Input: part model. Units: mm. Frame: model coordinates. A direction names the side the tool comes from. Round coordinates to 2 decimals unless told otherwise and drop trailing zeros. Write each loop counter-clockwise with the first axis right and the second up, starting at its lowest first coordinate (ties: lowest second). Pieces come first, ordered by that corner, then holes. Notation, with made-up numbers: (29.25, 63.25) -> (53.25, 63.25) arc R18 cw to (53.25, 73.25) -> close; hole circle Ø7 at (26, -17.5). An arc over 180 degrees is marked (long way). Write item = value, one per line.
```python
from build123d import *

# Parameters (mm, degrees)
SKETCH1_W                  = 38.1
SKETCH1_H                  = 88.9
BOSS_BASE_DEPTH            = 2.286
SKETCH3_W                  = 38.1
SKETCH3_H                  = 2.1717
BOSS_LIP_DEPTH             = 23.25116
F_4_0_209_DIAMETER_HOLE1_D = 5.3086
F_4_0_209_DIAMETER_HOLE2_D = 5.3086
SKETCH19_W                 = 4.445
SKETCH19_H                 = 66.04
CUT_EXTRUDE1_DEPTH         = 54.659308991
FILLET1_R                  = 3.81
FILLET4_R                  = 0.635


with BuildPart() as part:
    # Sketch1 → Boss-Base (new body)
    with BuildSketch(Plane(origin=(0, 0, 0), x_dir=(1, 0, 0), z_dir=(0, 1, 0))):
        Rectangle(SKETCH1_W, SKETCH1_H)
    extrude(amount=BOSS_BASE_DEPTH)

    # Sketch3 → Boss-Lip (add)
    with BuildSketch(Plane(origin=(0, 2.286, 0), x_dir=(1, 0, 0), z_dir=(0, 1, 0))):
        with Locations((0, 43.36415)):
            Rectangle(SKETCH3_W, SKETCH3_H)
    extrude(amount=BOSS_LIP_DEPTH)

    # #4 (0.209) Diameter Hole1 (through all)
    with Locations(Plane(origin=(0, 2.286, 0), x_dir=(1, 0, 0), z_dir=(0, 1, 0))):
        with Locations((0, -33.9217), (0, 6.7183)):
            Hole(F_4_0_209_DIAMETER_HOLE1_D / 2)

    # #4 (0.209) Diameter Hole2 (through all)
    with Locations(Plane.XY.offset(-42.2783)):
        with Locations((10.16, 17.78), (-10.16, 17.78)):
            Hole(F_4_0_209_DIAMETER_HOLE2_D / 2)

    # Sketch19 → Cut-Extrude1 (cut, through all)
    with BuildSketch(Plane(origin=(0, 2.286, 0), x_dir=(1, 0, 0), z_dir=(0, 1, 0))):
        with Locations((16.8275, -11.43)):
            Rectangle(SKETCH19_W, SKETCH19_H)
        with Locations((-16.8275, -11.43)):
            Rectangle(SKETCH19_W, SKETCH19_H)
    extrude(amount=-CUT_EXTRUDE1_DEPTH, mode=Mode.SUBTRACT)

    # Fillet1
    fillet1_edges = [part.edges().sort_by_distance(p)[0] for p in [
        (0, 2.286, -42.2783),
        (-19.05, 25.53716, -43.36415),
        (19.05, 25.53716, -43.36415),
        (0, 0, -44.45),
        (19.05, 1.143, -21.59),
        (14.605, 1.143, 44.45),
        (-19.05, 1.143, -21.59),
        (-14.605, 1.143, 44.45),
    ]]
    fillet(fillet1_edges, radius=FILLET1_R)

    # Fillet4
    fillet4_edges = [part.edges().sort_by_distance(p)[0] for p in [
        (19.05, 1.115923164, -43.334076836),
        (19.05, 3.401923164, -41.162376836),
        (-19.05, 3.401923164, -41.162376836),
        (14.605, 0, 9.525),
        (14.605, 2.286, 9.525),
        (-14.9225, 0, -21.59),
        (-14.9225, 2.286, -21.59),
        (19.05, 13.91158, -42.2783),
        (0, 25.53716, -42.2783),
        (-19.05, 13.91158, -42.2783),
        (17.934076836, 24.421236836, -42.2783),
        (-17.934076836, 24.421236836, -42.2783),
        (14.9225, 2.286, -21.59),
        (19.05, 2.286, -31.93415),
        (-19.05, 2.286, -31.93415),
        (-14.605, 2.286, 9.525),
        (0, 2.286, 44.45),
        (-17.934076836, 2.286, -22.705923164),
        (17.934076836, 2.286, -22.705923164),
        (13.489076836, 2.286, 43.334076836),
        (-13.489076836, 2.286, 43.334076836),
        (-19.05, 12.76858, -44.45),
        (0, 25.53716, -44.45),
        (19.05, 12.76858, -44.45),
        (17.934076836, 24.421236836, -44.45),
        (-17.934076836, 24.421236836, -44.45),
        (-19.05, 0, -33.02),
        (-19.05, 1.115923164, -43.334076836),
        (14.9225, 0, -21.59),
        (0, 0, 44.45),
        (-14.605, 0, 9.525),
        (19.05, 0, -33.02),
        (-17.934076836, 0, -22.705923164),
        (17.934076836, 0, -22.705923164),
        (13.489076836, 0, 43.334076836),
        (-13.489076836, 0, 43.334076836),
    ]]
    fillet(fillet4_edges, radius=FILLET4_R)


solid = part.part
```
1) Cut plane D-D (y = 7.25). Return the cut outline in (x, z) (3 decimals).
Solutions:
outline = (-19.05, -43.815) arc R0.635 ccw to (-18.415, -44.45) -> (18.415, -44.45) arc R0.635 ccw to (19.05, -43.815) -> (19.05, -42.913) arc R0.635 ccw to (18.415, -42.278) -> (-18.415, -42.278) arc R0.635 ccw to (-19.05, -42.913) -> close
2) First-contact query: P1, Ø0.5, axis at x = -15, y = 1.5, coming from the +Z side; P2, Ø0.5, axis at y = 1, z = 7.5, coming from the -X side (3 decimals); P3, Ø1.1, axis at y = 1.5, z = -2.5, coming from the +X side (3 decimals). Flat tips, straight axial feed; report the tip coordinate or a pass-through.
Solutions:
P1 = -21.59
P2 = -14.605
P3 = 14.605
3) Cut plane C-C (z = -33). Return the cut outline in (x, y) (3 decimals).
Solutions:
outline = (-19.05, 0.635) arc R0.635 ccw to (-18.415, 0) -> (18.415, 0) arc R0.635 ccw to (19.05, 0.635) -> (19.05, 1.651) arc R0.635 ccw to (18.415, 2.286) -> (-18.415, 2.286) arc R0.635 ccw to (-19.05, 1.651) -> close
4) Cut plane B-B (y = 17.78). Return the cut outline in (x, z) (3 decimals).
Solutions:
outline = (-19.05, -43.815) arc R0.635 ccw to (-18.415, -44.45) -> (-12.814, -44.45) -> (-12.814, -42.278) -> (-18.415, -42.278) arc R0.635 ccw to (-19.05, -42.913) -> close; (-7.506, -44.45) -> (7.506, -44.45) -> (7.506, -42.278) -> (-7.506, -42.278) -> close; (12.814, -44.45) -> (18.415, -44.45) arc R0.635 ccw to (19.05, -43.815) -> (19.05, -42.913) arc R0.635 ccw to (18.415, -42.278) -> (12.814, -42.278) -> close
5) Draft query along Z for faces 3 (the face through (-1.427, 1.127, -8.956)), 4 (the face through (0, 15, -42.278)), 5 (the face through (0, 0, 1)), 6 (the face through (0.58, 1.13, 36.51)). Return one class per face: +Z half, -Z half, draft (parallel to the pull), parting line (faces both ways), or undercut.
Solutions:
face_3 = undercut
face_4 = +Z half
face_5 = draft
face_6 = undercut
6) Line query: L1, parallel to Z at x = 0, y = 0.6; L2, parallel to Z at x = 0, y = 1.25; L3, parallel to Z at x = 4, y = 16.5. Output: solid intervals per line, ascending. Write a range as from..to.
Solutions:
L1 = -42.69..-9.37, -4.06..31.27, 36.58..44.45
L2 = -43.46..-9.37, -4.06..31.27, 36.58..44.45
L3 = -44.45..-42.28
7) Cut plane A-A (x = 0). Return the cut outline in (y, z) (3 decimals).
Solutions:
outline = (0, -40.64) arc R3.81 ccw to (3.81, -44.45) -> (24.902, -44.45) arc R0.635 ccw to (25.537, -43.815) -> (25.537, -42.913) arc R0.635 ccw to (24.902, -42.278) -> (6.096, -42.278) arc R3.81 cw to (2.286, -38.468) -> (2.286, -9.373) -> (0, -9.373) -> close; (0, -4.064) -> (2.286, -4.064) -> (2.286, 31.267) -> (0, 31.267) -> close; (0, 36.576) -> (2.286, 36.576) -> (2.286, 43.815) arc R0.635 ccw to (1.651, 44.45) -> (0.635, 44.45) arc R0.635 ccw to (0, 43.815) -> close
8) Access query for faces 1 (the face through (-13.459, 1.136, 43.364)), 2 (the face through (0, 2.286, 2)). Directions: +Z, -Z, +X, -X, +Y, -Y. A direction counts if a zero-diameter tool reaches every point of the face in a straight line with its end or side. Return the directions, or none.
Solutions:
face_1 = +Z, -X, +Y, -Y
face_2 = +Z, +X, -X, +Y
